Here's how the part is built. I have some questions about the finished solid (model axes, mm). Face numbers are marked on the shaded views. A direction names the side the tool comes from. Give positions to 0.01 mm unless a question says otherwise; leave off trailing zeros. Write each loop counter-clockwise with the first axis right and the second up, starting at its lowest first coordinate (ties: lowest second). Pieces come first, ordered by that corner, then holes. Notation, with made-up numbers: (45, 22.5) - (91, 22.5) arc R29 cw to (91, 43.5) - close; hole circle Ø8 at (4.5, 39). An arc over 180 degrees is marked (long way). Write each question's results on one line, items separated by ' | '. Start each with the question number.
Item 1: Which directions (+Z, -Z, +X, -X, +Y, -Y) give clear straight access to the entire face, cutting with the end or side of a thin tool? Please do the marked faces 1, 2, 3, 4 and 5.
Item 2: Will these pins go through, and if not, where does the flat tip stop? P1, Ø4.5, axis at x = -38.48, y = 33.93, coming from the +Z side; P2, Ø1.5, axis at y = 23.5, z = 13, coming from the -X side; P3, Ø3.5, axis at y = 23.5, z = 14, coming from the +X side.
Item 3: We'd pull the mould along Y, two halves only. Please class the marked faces 6, 7, 8 and 9: +Y half, -Y half, draft (parallel to the pull), parting line (faces both ways), or undercut.
Item 4: Suppose I cut it at D-D on z = 14. List the corners of the cut face in (x, y) for me.
Item 5: Suppose I cut it at C-C on y = 33. List the corners of the cut face in (x, z) for me.
Item 6: Suppose I cut it at A-A on x = -37.75. List the corners of the cut face in (y, z) for me, then the cut area to 3 significant figures.
Item 7: Please list where these lines run through material, in increasing order: line 1 along X through (y, z) = (33, 4.5); line 2 along X through (y, z) = (23.5, 8.25); line 3 along Z through (x, y) = (-51.5, 38).
Item 8: Suppose I cut it at B-B on z = 8.5. List the corners of the cut face in (x, y) for me.
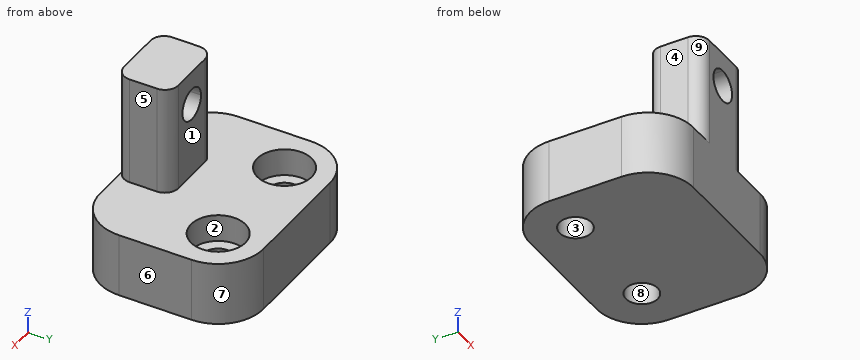
```python
from build123d import *

# Parameters (mm, degrees)
F0_R      = 3
F0_R_2    = 1.75
F1_DEPTH  = 7
F3_DEPTH  = 5
F4_W      = 8
F4_H      = 6
F5_DEPTH  = 12
F6_R      = 1.5
F2_R      = 3
F2_R_2    = 1.75
F7_DEPTH  = 3
F8_R      = 5
F10_DEPTH = 25


# Not quite as in the source:
# - a feature names something its author has since deleted; it is built from what else it names


with BuildPart() as f1:
    # F0 (on Top) → F1 (new body)
    with BuildSketch(Plane.XY):
        with BuildLine():
            ThreePointArc((-51.1365796847, 36.9232990628), (-48.9174910641, 36.1016771789), (-47.9842549264, 33.9271686971))
            ThreePointArc((-47.9842549264, 33.9271686971), (-50.9842549264, 30.9271686971), (-53.9842549264, 33.9271686971))
            Line((-53.9842549264, 33.9271686971), (-55.9842549264, 33.9271686971))
            Line((-55.9842549264, 33.9271686971), (-55.9842549264, 28.9271686971))
            Line((-55.9842549264, 28.9271686971), (-35.9842549264, 28.9271686971))
            Line((-35.9842549264, 28.9271686971), (-35.9842549264, 25.9271686971))
            Line((-35.9842549264, 25.9271686971), (-33.4842549264, 25.9271686971))
            Line((-33.4842549264, 25.9271686971), (-33.4842549264, 33.9271686971))
            Line((-33.4842549264, 33.9271686971), (-33.4842549264, 38.9232990628))
            Line((-33.4842549264, 38.9232990628), (-35.9842549264, 38.9232990628))
            Line((-35.9842549264, 38.9232990628), (-51.1365796847, 38.9232990628))
            Line((-51.1365796847, 38.9232990628), (-51.1365796847, 36.9232990628))
        make_face()
        with Locations((-38.4842549264, 33.9271686971)):
            Circle(F0_R, mode=Mode.SUBTRACT)
        with BuildLine():
            ThreePointArc((-53.9842549264, 33.9271686971), (-53.1587634082, 35.9939325595), (-51.1365796847, 36.9232990628))
            Line((-51.1365796847, 36.9232990628), (-51.1365796847, 38.9232990628))
            Line((-51.1365796847, 38.9232990628), (-55.9842549264, 38.9232990628))
            Line((-55.9842549264, 38.9232990628), (-55.9842549264, 33.9271686971))
            Line((-55.9842549264, 33.9271686971), (-53.9842549264, 33.9271686971))
        make_face()
        Polygon((-35.9842549264, 28.9271686971), (-55.9842549264, 28.9271686971), (-55.9842549264, 25.9271686971), (-53.9842549264, 25.9271686971), (-43.9842549264, 25.9271686971), (-35.9842549264, 25.9271686971), align=None)
        with BuildLine():
            ThreePointArc((-53.9842549264, 33.9271686971), (-50.9842549264, 30.9271686971), (-47.9842549264, 33.9271686971))
            ThreePointArc((-47.9842549264, 33.9271686971), (-48.9174910641, 36.1016771789), (-51.1365796847, 36.9232990628))
            ThreePointArc((-51.1365796847, 36.9232990628), (-53.1587634082, 35.9939325595), (-53.9842549264, 33.9271686971))
        make_face()
        with Locations((-50.9842549264, 33.9271686971)):
            Circle(F0_R_2, mode=Mode.SUBTRACT)
        with Locations((-38.4842549264, 33.9271686971)):
            Circle(F0_R)
        with Locations((-38.4842549264, 33.9271686971)):
            Circle(F0_R_2, mode=Mode.SUBTRACT)
    extrude(amount=F1_DEPTH)

    # F3 (add): a face of the model
    f3_faces = [f1.faces().sort_by_distance(p)[0] for p in [
        (-44.7342549264, 25.9271686971, 3.5),
    ]]
    extrude(f3_faces, amount=F3_DEPTH)

    # F4 (on face) → F5 (join)
    with BuildSketch(Plane.XY.offset(7)):
        with Locations((-45.4842549264, 23.9271686971)):
            Rectangle(F4_W, F4_H)
    extrude(amount=F5_DEPTH)

    # F6
    f6_edges = [f1.edges().sort_by_distance(p)[0] for p in [
        (-49.484255, 20.927169, 13),
        (-41.484255, 20.927169, 13),
        (-49.484255, 26.927169, 13),
        (-41.484255, 26.927169, 13),
    ]]
    fillet(f6_edges, radius=F6_R)

    # F2 (on face) → F7 (cut)
    with BuildSketch(Plane.XY.offset(7)):
        with Locations((-50.9842549264, 33.9271686971)):
            Circle(F2_R)
        with Locations((-50.9842549264, 33.9271686971)):
            Circle(F2_R_2, mode=Mode.SUBTRACT)
        with Locations((-38.4842549264, 33.9271686971)):
            Circle(F2_R)
        with Locations((-38.4842549264, 33.9271686971)):
            Circle(F2_R_2, mode=Mode.SUBTRACT)
    extrude(amount=-F7_DEPTH, mode=Mode.SUBTRACT)

    # F8
    f8_edges = [f1.edges().sort_by_distance(p)[0] for p in [
        (-55.984255, 20.927169, 3.5),
        (-55.984255, 38.923299, 3.5),
        (-33.484255, 38.923299, 3.5),
        (-33.484255, 20.927169, 3.5),
    ]]
    fillet(f8_edges, radius=F8_R)

    # F9 (on face) → F10 (cut)
    with BuildSketch(Plane(origin=(0, 26.9271686971, 0), x_dir=(-1, 0, 0), z_dir=(0, 1, 0))):
        with BuildLine():
            ThreePointArc((45.4842549264, 17), (44.2468180594, 14.0125631329), (47.2342549264, 15.25))
            ThreePointArc((47.2342549264, 15.25), (46.7216917935, 16.4874368671), (45.4842549264, 17))
        make_face()
    extrude(amount=-F10_DEPTH, mode=Mode.SUBTRACT)


solid = f1.part
```
Checked values:
1) face 1: +Z, +X, -X, +Y | face 2: +Z | face 3: +Z, -Z | face 4: +Z, -X, +Y, -Y | face 5: +Z, +X, +Y, -Y
2) P1: stops at z = 4 | P2: stops at x = -49.48 | P3: stops at x = -41.48
3) face 6: draft | face 7: +Y half | face 8: undercut | face 9: -Y half
4) outline: (-49.48, 22.43) arc R1.5 ccw to (-47.98, 20.93) - (-46.71, 20.93) - (-46.71, 26.93) - (-47.98, 26.93) arc R1.5 ccw to (-49.48, 25.43) - close; (-44.26, 20.93) - (-42.98, 20.93) arc R1.5 ccw to (-41.48, 22.43) - (-41.48, 25.43) arc R1.5 ccw to (-42.98, 26.93) - (-44.26, 26.93) - close
5) outline: (-55.98, 0) - (-52.47, 0) - (-52.47, 4) - (-53.84, 4) - (-53.84, 7) - (-55.98, 7) - close; (-49.5, 0) - (-39.97, 0) - (-39.97, 4) - (-41.34, 4) - (-41.34, 7) - (-48.13, 7) - (-48.13, 4) - (-49.5, 4) - close; (-37, 0) - (-33.48, 0) - (-33.48, 7) - (-35.63, 7) - (-35.63, 4) - (-37, 4) - close
6) outline: (20.98, 0) - (32.34, 0) - (32.34, 4) - (31.02, 4) - (31.02, 7) - (20.98, 7) - close; (35.52, 0) - (38.87, 0) - (38.87, 7) - (36.84, 7) - (36.84, 4) - (35.52, 4) - close | area: 95.1 mm^2
7) line 1: x = -55.98 to -53.84, -48.13 to -41.34, -35.63 to -33.48 | line 2: x = -49.48 to -41.48 | line 3: z = 0 to 7
8) outline: (-49.48, 22.43) arc R1.5 ccw to (-47.98, 20.93) - (-42.98, 20.93) arc R1.5 ccw to (-41.48, 22.43) - (-41.48, 25.43) arc R1.5 ccw to (-42.98, 26.93) - (-47.98, 26.93) arc R1.5 ccw to (-49.48, 25.43) - close
